from build123d import *

# Parameters (mm, degrees)
F0_R          = 9.5
F1_DEPTH      = 17.5
F1_DEPTH_BACK = 17.5
F2_R          = 2.15
F3_DEPTH      = 25
F4_SIZE       = 0.5
F5_R          = 9.5
F5_R_2        = 8.5
F6_DEPTH      = 2
F8_R          = 10
F9_DEPTH      = 1
F10_SIZE      = 0.5
F11_SIZE      = 0.5
F12_SIZE      = 0.5


with BuildPart() as f1:
    # F0 (on Top) → F1 (new body, two sides)
    with BuildSketch(Plane.XY) as f1_sk:
        Polygon((8, -13), (19, -13), (20, -12), (20, -5), (19, -3), (19, 6.723037264), (18, 8), (10, 8), (6, 13), (-6, 13), (-10, 8), (-18, 8), (-19, 6.723037264), (-19, -3), (-20, -5), (-20, -12), (-19, -13), (-8, -13), (-7, -12.5), (7, -12.5), align=None)
        Circle(F0_R, mode=Mode.SUBTRACT)
    extrude(amount=F1_DEPTH)
    extrude(f1_sk.sketch, amount=-F1_DEPTH_BACK)

    # F2 (on face) → F3 (cut)
    with BuildSketch(Plane.XZ.offset(13)):
        with Locations((-14, 10.5)):
            Circle(F2_R)
        with Locations((14, 10.5)):
            Circle(F2_R)
        with Locations((14, -10.5)):
            Circle(F2_R)
        with Locations((-14, -10.5)):
            Circle(F2_R)
    extrude(amount=-F3_DEPTH, mode=Mode.SUBTRACT)

    # F4
    f4_edges = [f1.edges().sort_by_distance(p)[0] for p in [
        (-16.15, 8, 10.5),
        (-16.15, 8, -10.5),
        (11.85, 8, -10.5),
        (11.85, 8, 10.5),
        (-16.15, -13, 10.5),
        (-16.15, -13, -10.5),
        (11.85, -13, -10.5),
        (11.85, -13, 10.5),
    ]]
    chamfer(f4_edges, length=F4_SIZE)

    # F5 (on face) → F6 (join)
    with BuildSketch(Plane(origin=(0, 0, -17.5), x_dir=(1, 0, 0), z_dir=(0, 0, -1))):
        Circle(F5_R)
        Circle(F5_R_2, mode=Mode.SUBTRACT)
    extrude(amount=-F6_DEPTH)

    # F8 (on offset) → F9 (cut)
    with BuildSketch(Plane.XY.offset(15.5)):
        Circle(F8_R)
    extrude(amount=-F9_DEPTH, mode=Mode.SUBTRACT)

    # F10
    f10_edges = [f1.edges().sort_by_distance(p)[0] for p in [
        (-10, 8, 0),
        (-6, 13, 0),
        (6, 13, 0),
        (10, 8, 0),
    ]]
    chamfer(f10_edges, length=F10_SIZE)

    # F11
    f11_edges = [f1.edges().sort_by_distance(p)[0] for p in [
        (14.25, 8, 17.5),
        (10.093826, 8.195217, 17.5),
        (18.5, 7.361519, 17.5),
        (8, 10.5, 17.5),
        (19, 1.861519, 17.5),
        (5.906174, 12.804783, 17.5),
        (19.5, -4, 17.5),
        (0, 13, 17.5),
        (20, -8.5, 17.5),
        (-5.906174, 12.804783, 17.5),
        (19.5, -12.5, 17.5),
        (-8, 10.5, 17.5),
        (13.5, -13, 17.5),
        (-10.093826, 8.195217, 17.5),
        (7.5, -12.75, 17.5),
        (-14.25, 8, 17.5),
        (0, -12.5, 17.5),
        (-18.5, 7.361519, 17.5),
        (-7.5, -12.75, 17.5),
        (-19, 1.861519, 17.5),
        (-13.5, -13, 17.5),
        (-19.5, -4, 17.5),
        (-19.5, -12.5, 17.5),
        (-20, -8.5, 17.5),
        (-9.5, 0, 17.5),
    ]]
    chamfer(f11_edges, length=F11_SIZE)

    # F12
    f12_edges = [f1.edges().sort_by_distance(p)[0] for p in [
        (14.25, 8, -17.5),
        (10.093826, 8.195217, -17.5),
        (18.5, 7.361519, -17.5),
        (8, 10.5, -17.5),
        (19, 1.861519, -17.5),
        (5.906174, 12.804783, -17.5),
        (19.5, -4, -17.5),
        (0, 13, -17.5),
        (20, -8.5, -17.5),
        (-5.906174, 12.804783, -17.5),
        (19.5, -12.5, -17.5),
        (-8, 10.5, -17.5),
        (13.5, -13, -17.5),
        (-10.093826, 8.195217, -17.5),
        (7.5, -12.75, -17.5),
        (-14.25, 8, -17.5),
        (0, -12.5, -17.5),
        (-18.5, 7.361519, -17.5),
        (-7.5, -12.75, -17.5),
        (-19, 1.861519, -17.5),
        (-13.5, -13, -17.5),
        (-19.5, -4, -17.5),
        (-19.5, -12.5, -17.5),
        (-20, -8.5, -17.5),
        (-8.5, 0, -17.5),
    ]]
    chamfer(f12_edges, length=F12_SIZE)


solid = f1.part
Read the model definition and answer for the solid it produces. Units are mm, in the model's axes. A direction names the side the tool comes from. Give positions to 0.01 mm unless a question says otherwise; leave off trailing zeros. Write each loop counter-clockwise with the first axis right and the second up, starting at its lowest first coordinate (ties: lowest second). Pieces come first, ordered by that corner, then holes. Notation, with made-up numbers: (26.25, -26.5) - (57.25, -26.5) arc R13 ccw to (57.25, -20.5) - close; hole circle Ø2 at (-36.5, 73). An arc over 180 degrees is marked (long way). Answer in a Markdown table with one row per item. Add a question column.
Item 1: Section A-A, the plane y = 0 is taken. Count the separate pieces of the cut face and the enclosed holes in it, and give its area (3 significant figures).
Item 2: Determine the mould class of faces 1 (the face through (19.26, -4.072, 17.246)), 2 (the face through (4.57, -7.167, -16.26)), 3 (the face through (-2.17, -9.76, 15.01)) for opening direction Z: pulls with the +Z half, pulls with the -Z half, needs draft (parallel to the pull), parting line crosses it, or undercut.
Item 3: Flat-ended cylindrical pins translate along their axes: P1, Ø10.5, axis at y = 3.5, z = -1, coming from the +X side; P2, Ø12, axis at x = -12.5, z = -12, coming from the +Y side (3 decimals); P3, Ø3, axis at y = 3.5, z = 2.5, coming from the -X side; P4, Ø11.5, axis at x = 0, y = 0, coming from the +Z side. Find the tip coordinate at first contact, or state that the pin passes through.
Item 4: Section C-C, the plane z = -4.5 is taken. Write down the section's boundary in (x, y).
Item 5: A tool of negligible diameter and unlimited length cuts with its end or side. For faces 4 (the face through (20, -9, 0)), 5 (the face through (-7.568, -12.501, -17.254)), from which of +Z, -Z, +X, -X, +Y, -Y can it reach the whole face along a straight path? Write none if from no direction.
Item 6: Section B-B, the plane x = 14 is taken. Write down the section's boundary in (y, z).
Item 7: Find the intervals of material crossed by L1, parallel to Z at x = -14, y = 0; L2, parallel to X at y = 0, z = 16.2; L3, parallel to X at y = -1.5, z = -11.5, in increasing order.
Recorded:
| question | item | result |
|---|---|---|
| 1 | separate pieces | 2 |
| 1 | enclosed holes | 4 |
| 1 | area | 609 mm2 |
| 2 | face 1 | pulls with the +Z half |
| 2 | face 2 | needs draft |
| 2 | face 3 | undercut |
| 3 | P1 | stops at x = 19 |
| 3 | P2 | stops at y = 12.375 |
| 3 | P3 | stops at x = -19 |
| 3 | P4 | passes through |
| 4 | outline | (-20, -12) - (-19, -13) - (-8, -13) - (-7, -12.5) - (7, -12.5) - (8, -13) - (19, -13) - (20, -12) - (20, -5) - (19, -3) - (19, 6.72) - (18, 8) - (10.5, 8) - (9.69, 8.39) - (6.31, 12.61) - (5.5, 13) - (-5.5, 13) - (-6.31, 12.61) - (-9.69, 8.39) - (-10.5, 8) - (-18, 8) - (-19, 6.72) - (-19, -3) - (-20, -5) - close; hole circle Ø19 at (0, 0) |
| 5 | face 4 | +Z, -Z, +X, +Y, -Y |
| 5 | face 5 | -Z, -Y |
| 6 | outline | (-13, -17) - (-12.5, -17.5) - (7.5, -17.5) - (8, -17) - (8, -13.15) - (7.5, -12.65) - (-12.5, -12.65) - (-13, -13.15) - close; (-13, -7.85) - (-12.5, -8.35) - (7.5, -8.35) - (8, -7.85) - (8, 7.85) - (7.5, 8.35) - (-12.5, 8.35) - (-13, 7.85) - close; (-13, 13.15) - (-12.5, 12.65) - (7.5, 12.65) - (8, 13.15) - (8, 17) - (7.5, 17.5) - (-12.5, 17.5) - (-13, 17) - close |
| 7 | L1 | z = -17.5 to -12.65, -8.35 to 8.35, 12.65 to 17.5 |
| 7 | L2 | x = -19 to -9.5, 9.5 to 19 |
| 7 | L3 | x = -19 to -15.9, -12.1 to -9.38, 9.38 to 12.1, 15.9 to 19 |
